Can you work these out from the model? Positions are in its coordinate system, mm. Face numbers are marked on the shaded views. Round coordinates to 2 decimals unless told otherwise and drop trailing zeros. Loops run counter-clockwise (first coordinate to the right, second up) from the corner with the lowest first, then second, coordinate; pieces in that order, holes last.
(1) Thinking about a two-plate mould opening in Z: for the marked faces 1, 2 and 3, which applies, released by +Z, released by -Z, zero draft, split by the parting line, or undercut?
(2) I want a section at C-C on z = -2.5. Write out the boundary of the cut face in (x, y), plus the area to 3 significant figures.
(3) I want a section at B-B on x = 7.25. Write out the boundary of the cut face in (y, z).
(4) I want a section at A-A on x = 5.15. Write out the boundary of the cut face in (y, z), plus the area to 3 significant figures.
(5) I want a section at D-D on y = -13.75. Write out the boundary of the cut face in (x, z), plus the area to 3 significant figures.
(6) Will this pin go through, and if not, where does the flat tip stop? pin 1 Ø1 at (x, z) = (4.5, -1) entering from -Y.
(7) If I drill on line 1 along Z through (x, y) = (5.2, -7.5); line 2 along Z through (x, y) = (5.7, -7.25); line 3 along Z through (x, y) = (6, -12.75), over which ranges is the centre line in solid material (lowest first)?
Autodesk Inventor part; units mm, degrees
ref_plane "YZ Plane" through (0, 0, 0) normal (1, 0, 0) x (0, 1, 0)
ref_plane "XZ Plane" through (0, 0, 0) normal (0, 1, 0) x (-1, 0, 0)
ref_plane "XY Plane" through (0, 0, 0) normal (0, 0, 1) x (1, 0, 0)
sketch "Sketch1" plane through (0, 0, 0) normal (1, 0, 0) x (0, 1, 0)
  arc A0 (-1.2115, 27.4733) -> (-1.2115, -27.4733) centre (0, 0) ccw
  line L0 (-1.2115, -27.4733) -> (-6.2115, -27.4733)
  line L1 (-6.2115, -27.4733) -> (-6.2115, 27.4733)
  line L2 (-6.2115, 27.4733) -> (-1.2115, 27.4733)
  line L3 (-6.2115, -26.7893) -> (-6.2115, 26.7893)
  line L4 (-6.2115, 0) -> (-6.2115, 26.7893)
  circle A1 centre (0, 0) radius 27.5
  point P0 (5.2115, 24.6247)
  dimension "d0" = 5
  dimension "d1" = 53.5786
extrude "Extrusion1" add sketch "Sketch1" along normal blind 7.5 contours L1 A0
sketch "Sketch2" plane through (0, -6.2115, 26.7893) normal (0, 1, 0) x (1, 0, 0)
  line L0 (0, 6.9167) -> (7.5, 6.9167)
  line L1 (0, 0) -> (0, 6.9167)
  line L2 (0, 6.9167) -> (7.5, 6.9167)
  line L3 (7.5, 26.7893) -> (7.5, 0)
  line L4 (7.5, 6.9167) -> (7.5, 0)
  line L5 (7.5, 0) -> (0, 0)
  line L6 (7.5, 0) -> (0, 0)
  circle A0 centre (3.75, 3.4583) radius 1
  line L7 (0, 0) -> (0, 53.5786)
  line L8 (0, 53.5786) -> (0, 0)
  line L9 (0, 26.7893) -> (7.5, 26.7893)
  circle A1 centre (3.75, 50.1203) radius 1
  circle A2 centre (3.75, 3.4583) radius 2
  circle A3 centre (3.75, 50.1203) radius 2
  line L10 (0, 6.9167) -> (7.5, 6.9167)
  line L11 (0, 0) -> (0, 6.9167)
  line L12 (0, 6.9167) -> (7.5, 6.9167)
  line L13 (7.5, 26.7893) -> (7.5, 0)
  line L14 (7.5, 6.9167) -> (7.5, 0)
  line L15 (7.5, 0) -> (0, 0)
  line L16 (7.5, 0) -> (0, 0)
  line L17 (0, 0) -> (2.2798, 2.1025)
  line L18 (5.2202, 4.8142) -> (7.5, 6.9167)
  line L19 (0, 6.9167) -> (2.2798, 4.8142)
  line L20 (5.2202, 2.1025) -> (7.5, 0)
  line L21 (0, 0) -> (0, 53.5786)
  line L22 (0, 53.5786) -> (0, 0)
  line L23 (0, 26.7893) -> (7.5, 26.7893)
  circle A4 centre (3.75, 50.1203) radius 1
  line L24 (0, 53.5786) -> (7.5, 53.5786)
  line L25 (7.5, 53.5786) -> (7.5, 0)
  circle A5 centre (3.75, 50.1203) radius 2
  circle A6 centre (3.75, 3.4583) radius 2
  point P0 (0, 26.7893)
  point P1 (280.32, 51.414)
  point P2 (4.4851, 4.1363)
  point P3 (4.4851, 2.7804)
  point P4 (3.0149, 4.1363)
  point P5 (3.0149, 2.7804)
  point P6 (280.32, 51.414)
  dimension "d6" = 2
  dimension "d9" = 4
  dimension "d10" = 4
  dimension "d13" = 4
  dimension "d14" = 4
extrude "Extrusion2" cut sketch "Sketch2" against normal blind 10 contours A0 | A1
extrude "Extrusion3" cut sketch "Sketch2" against normal blind 13.175 contours A2 | A3
scale "Scale1" factors (0.5, 0.5, 0.5) then translate (3.75, -3.1057, 0) bodies 1
properties part number "Contrapeso1"
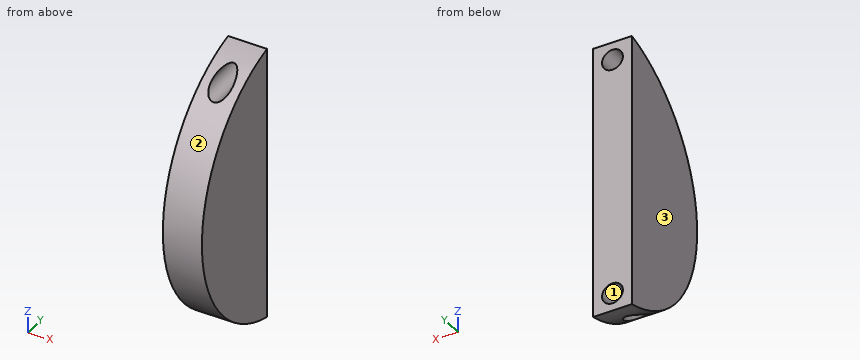
Filled sheet:
1. face 1: undercut
1. face 2: split by the parting line
1. face 3: zero draft
2. outline: (3.75, -16.63) - (7.5, -16.63) - (7.5, -6.21) - (3.75, -6.21) - close
2. area: 39.1 mm2
3. outline: (-6.21, -13.39) - (-6.21, 13.39) arc R13.75 ccw to start
4. outline: (-11.63, -10.79) - (-6.21, -10.79) - (-6.21, 10.79) - (-11.63, 10.79) arc R13.75 ccw to start; (-8.73, -12.55) arc R13.75 ccw to (-6.21, -13.39) - (-6.21, -12.55) - close; (-8.73, 12.55) - (-6.21, 12.55) - (-6.21, 13.39) arc R13.75 ccw to start
4. area: 198 mm2
5. outline: (3.75, -8.7) - (7.5, -8.7) - (7.5, 8.7) - (3.75, 8.7) - close
5. area: 65.3 mm2
6. pin 1: stops at y = -16.85
7. line 1: z = -13.03 to -12.57, -10.76 to 10.76, 12.57 to 13.03
7. line 2: z = -13.11 to -12.66, -10.67 to 10.67, 12.66 to 13.11
7. line 3: z = -9.8 to 9.8
